Can you work these out from the model? Positions are in its coordinate system, mm. A direction names the side the tool comes from. Coordinates: 2 decimals unless noted, no trailing zeros. Order: outer loops, then holes, each group sorted by start corner. A loop starts at its lowest first (then second) coordinate and runs counter-clockwise, first axis right, second up.
```python
from build123d import *

# Parameters (mm, degrees)
BOSS_EXTRU_1_DEPTH           = 75
ESQUISSE3_R                  = 15
BOSS_EXTRU_2_DEPTH           = 162.5
BOSS_EXTRU_3_START           = 162.5
ESQUISSE4_R                  = 15
BOSS_EXTRU_3_DEPTH           = 162.5
ESQUISSE5_W                  = 15
ESQUISSE5_H                  = 15
R_P_TITION_CIRCULAIRE2_COUNT = 3


with BuildPart() as part:
    # Esquisse1 → Boss.-Extru.1 (new body)
    with BuildSketch(Plane.XY):
        Polygon((-20.36542333, 6.148938206), (-57.86542333, -58.802967077), (17.13457667, -58.802967077), align=None)
    extrude(amount=BOSS_EXTRU_1_DEPTH)

    # Esquisse3 → Boss.-Extru.2 (add)
    with BuildSketch(Plane.XY.offset(75)):
        with Locations((-20.36542333, -37.152331983)):
            Circle(ESQUISSE3_R)
    extrude(amount=BOSS_EXTRU_2_DEPTH)

    # Esquisse4 → Boss.-Extru.3 (add)
    with BuildSketch(Plane(origin=(0, 0, 0), x_dir=(-1, 0, 0), z_dir=(0, 0, -1)).offset(BOSS_EXTRU_3_START)):
        with Locations(Location((20.36542333, -37.152331983, 0), (0, 0, 180))):
            Circle(ESQUISSE4_R)
    extrude(amount=-BOSS_EXTRU_3_DEPTH)

    # Balayage1: sweep along a curve in space
    with BuildLine() as balayage1_path:
        Line((-12.950526791, -56.834039487, 37.5), (-12.950526791, -79.630989253, 37.5))
        Line((-12.950526791, -79.630989253, 37.5), (-32.950526791, -79.630989253, 37.5))
        Line((-32.950526791, -79.630989253, 37.5), (-32.950526791, -157.328083579, 37.5))
        Line((-32.950526791, -157.328083579, 37.5), (-22.950526791, -157.328083579, 37.5))
    # Esquisse5 → Balayage1 (sweep)
    with BuildSketch(Plane.XZ.offset(58.802967077)):
        with Locations((-20.36542333, 37.5)):
            Rectangle(ESQUISSE5_W, ESQUISSE5_H)
    balayage1 = sweep(path=balayage1_path.line, transition=Transition.RIGHT)

    # Répétition circulaire2: Balayage1 ×3 about axis
    r_p_tition_circulaire2_axis = Axis((-20.36542333, -37.152331983, 0), (0, 0, 1))
    for i in range(1, R_P_TITION_CIRCULAIRE2_COUNT):
        add(balayage1.rotate(r_p_tition_circulaire2_axis, i * 360 / R_P_TITION_CIRCULAIRE2_COUNT))


solid = part.part
```
1. Please list where these lines run through material, in increasing order: probe 1 along X at (y, z) = (-9, 42); probe 2 along X at (y, z) = (-38.5, -142); probe 3 along X at (y, z) = (-126, 43.5).
Completed:
probe 1: x = -53.26 to -35.94, -29.11 to -11.62, 53.4 to 83.4
probe 2: x = -35.3 to -5.43
probe 3: x = -47.87 to -32.87
2. Imagine slicing it at C-C on x = 31.5. Please give me the cut outline in (y, z).
Completed:
outline: (-38.96, 30) - (-21.64, 30) - (-21.64, 45) - (-38.96, 45) - close
3. Thinking about a two-plate mould opening in X: for faces 6 (the flat face through (-28, -157.243, 37)), 7 (the flat face through (3.82, -14.53, 37.4)), 8 (the flat face through (-120.63, 29.365, 37.395)), 9 (the cylindrical face through (-23.62, -22.51, -82.39)), which applies, pulls with the +X half, pulls with the -X half, needs draft (parallel to the pull), parting line crosses it, or undercut?
Completed:
face 6: needs draft
face 7: undercut
face 8: undercut
face 9: parting line crosses it
4. On a 3-axis mill with a long thin cutter (end or side, diameter ignored), from which of +Z, -Z, +X, -X, +Y, -Y can I reach the whole of each face in a straight line? I mean faces 1 (the flat face through (12.3, -38.6, 37.6)), 2 (the flat face through (44, -16, 30)), 3 (the flat face through (-23, -79.716, 37)), 4 (the flat face through (91.515, 24.457, 37.395)), 5 (the flat face through (-32, -48, 75)). Say none if no direction works.
Completed:
face 1: +Z, -Z
face 2: -Z, +X, +Y
face 3: +Z, -Z, +X
face 4: +Z, -Z, +Y
face 5: +Z
5. Imagine slicing it at D-D on z = 199.5. Please give me the cut outline in (x, y), then the cut area to 3 significant figures.
Completed:
outline: circle Ø30 at (-20.37, -37.15)
area: 707 mm2
6. Imagine slicing it at B-B on y = -131.5. Please give me the cut outline in (x, z).
Completed:
outline: (-47.87, 30) - (-32.87, 30) - (-32.87, 45) - (-47.87, 45) - close
7. I'm going to push flat-ended pins straight in: pin 1 (2 mm diameter, centred on y = -23.5, z = 106.5, fed in from +X); pin 2 (7.5 mm diameter, centred on y = -133, z = 34.5, fed in from +X); pin 3 (12 mm diameter, centred on y = -68, z = 40, fed in from +X). Where does each tip first touch, or does it pass through?
Completed:
pin 1: stops at x = -12.31
pin 2: stops at x = -32.87
pin 3: stops at x = -12.87
8. Imagine slicing it at A-A on z = 62.5. Please give me the cut outline in (x, y).
Completed:
outline: (-57.87, -58.8) - (17.13, -58.8) - (-20.37, 6.15) - close
